Could you check a few things on this model? Use its own coordinates, in mm. Face numbers are marked on the shaded views. A direction names the side the tool comes from. Coordinates: 2 decimals unless noted, no trailing zeros. Order: outer loops, then holes, each group sorted by start corner. A loop starts at its lowest first (then second) coordinate and runs counter-clockwise, first axis right, second up. Notation, with made-up numbers: (88, 76.25) - (107, 76.25) arc R33 ccw to (107, 112.25) - close; hole circle Ø7 at (-0.75, 17). An arc over 180 degrees is marked (long way). Answer as a JSON object with one key per item and string values. Group by question number.
(1) Imagine slicing it at D-D, the plane y = -26.5. Write out the boundary of the cut face in (x, z).
(2) Imagine slicing it at B-B, the plane z = 4.75. Write out the boundary of the cut face in (x, y).
(3) Will these pins go through, and if not, where does the flat tip stop? P1, Ø1.5, axis at x = 68, z = 5.5, coming from the +Y side; P2, Ø2.5, axis at y = -10, z = 3, coming from the -X side; P3, Ø3, axis at y = -25.5, z = 6, coming from the -X side; P4, Ø2.5, axis at x = 75, z = 4, coming from the -Y side.
(4) Imagine slicing it at C-C, the plane x = 35. Write out the boundary of the cut face in (y, z), and give its area (3 significant figures).
(5) We'd pull the mould along X, two halves only. Please class the marked faces 1, 2, 3 and 4: pulls with the +X half, pulls with the -X half, needs draft (parallel to the pull), parting line crosses it, or undercut.
(6) Imagine slicing it at A-A, the plane y = -19.5. Write out the boundary of the cut face in (x, z).
(7) Which directions (+Z, -Z, +X, -X, +Y, -Y) give clear straight access to the entire face, cutting with the end or side of a thin tool? Please do the marked faces 5 and 6.
(8) Please list where these lines run through material, in increasing order: probe 1 along X at (y, z) = (-4, 4.75); probe 2 along X at (y, z) = (-12.5, 2); probe 3 along Y at (x, z) = (30.5, 2.25).
from build123d import *

# Parameters (mm, degrees)
BOSS_EXTRU_1_DEPTH      = 7.5
ESQUISSE2_R             = 1.6
ENL_V_MAT_EXTRU_1_DEPTH = 83.050289457
CHANFREIN1_SIZE         = 8
CHANFREIN1_SIZE2        = 17.156055364
CHANFREIN2_SIZE         = 5
CHANFREIN2_SIZE2        = 10.722534603
ESQUISSE3_W             = 3
ESQUISSE3_H             = 6
ESQUISSE3_H_2           = 5
ENL_V_MAT_EXTRU_2_DEPTH = 83.050289457


with BuildPart() as part:
    # Esquisse1 → Boss.-Extru.1 (new body)
    with BuildSketch(Plane.XY):
        Polygon((0, 0), (0, -30), (76, -30), (76, 0), (55, 0), (55, -23), (14.5, -23), (14.5, 0), align=None)
    extrude(amount=BOSS_EXTRU_1_DEPTH)

    # Esquisse2 → Enlèv. mat.-Extru.1 (cut, through all)
    with BuildSketch(Plane(origin=(0, 0, 0), x_dir=(-1, 0, 0), z_dir=(0, 0, -1))):
        with Locations((-11.746558558, -16.576326178)):
            Circle(ESQUISSE2_R)
        with Locations((-11.746558558, -6.348778822)):
            Circle(ESQUISSE2_R)
        with Locations((-58.966054895, -16.576326178)):
            Circle(ESQUISSE2_R)
        with Locations((-58.966054895, -6.348778822)):
            Circle(ESQUISSE2_R)
    extrude(amount=-ENL_V_MAT_EXTRU_1_DEPTH, mode=Mode.SUBTRACT)

    # Chanfrein1
    chanfrein1_edges = [part.edges().sort_by_distance(p)[0] for p in [
        (0, -30, 3.75),
    ]]
    chanfrein1_side = [part.faces().sort_by_distance(p)[0] for p in [
        (0, -15, 3.75),
    ]]
    chamfer(chanfrein1_edges, length=CHANFREIN1_SIZE, length2=CHANFREIN1_SIZE2, reference=chanfrein1_side[0])

    # Chanfrein2
    chanfrein2_edges = [part.edges().sort_by_distance(p)[0] for p in [
        (76, -30, 3.75),
    ]]
    chanfrein2_side = [part.faces().sort_by_distance(p)[0] for p in [
        (76, -15, 3.75),
    ]]
    chamfer(chanfrein2_edges, length=CHANFREIN2_SIZE, length2=CHANFREIN2_SIZE2, reference=chanfrein2_side[0])

    # Esquisse3 → Enlèv. mat.-Extru.2 (cut, through all)
    with BuildSketch(Plane.XY.offset(7.5)):
        with Locations((74.5, -11)):
            Rectangle(ESQUISSE3_W, ESQUISSE3_H)
        with Locations((1.5, -9.5)):
            Rectangle(ESQUISSE3_W, ESQUISSE3_H_2)
    extrude(amount=-ENL_V_MAT_EXTRU_2_DEPTH, mode=Mode.SUBTRACT)


solid = part.part
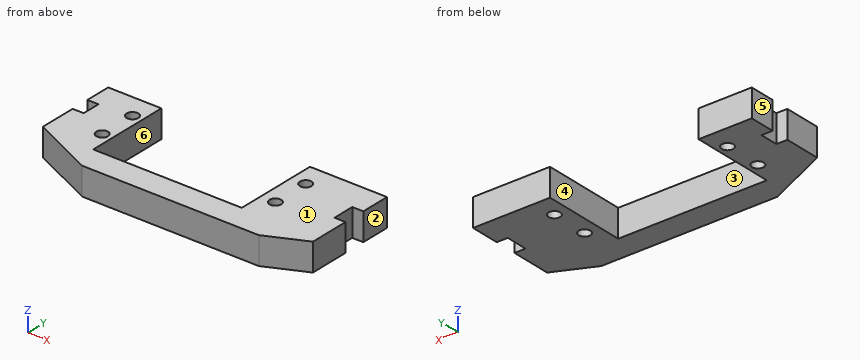
Result set:
{
 "1": {"outline": "(9.65, 0) - (72.78, 0) - (72.78, 7.5) - (9.65, 7.5) - close"},
 "2": {"outline": "(0, -22) - (17.16, -30) - (65.28, -30) - (76, -25) - (76, -14) - (73, -14) - (73, -8) - (76, -8) - (76, 0) - (55, 0) - (55, -23) - (14.5, -23) - (14.5, 0) - (0, 0) - (0, -7) - (3, -7) - (3, -12) - (0, -12) - close; hole circle Ø3.2 at (11.75, -16.58); hole circle Ø3.2 at (11.75, -6.35); hole circle Ø3.2 at (58.97, -16.58); hole circle Ø3.2 at (58.97, -6.35)"},
 "3": {"P1": "stops at y = 0", "P2": "stops at x = 3", "P3": "stops at x = 4.29", "P4": "stops at y = -26.05"},
 "4": {"outline": "(-30, 0) - (-23, 0) - (-23, 7.5) - (-30, 7.5) - close", "area": "52.5 mm^2"},
 "5": {"face 1": "needs draft", "face 2": "pulls with the +X half", "face 3": "undercut", "face 4": "undercut"},
 "6": {"outline": "(0, 0) - (14.5, 0) - (14.5, 7.5) - (0, 7.5) - close; (55, 0) - (76, 0) - (76, 7.5) - (55, 7.5) - close"},
 "7": {"face 5": "+Z, -Z, -X, +Y, -Y", "face 6": "+Z, -Z, +Y"},
 "8": {"probe 1": "x = 0 to 14.5, 55 to 76", "probe 2": "x = 0 to 14.5, 55 to 73", "probe 3": "y = -30 to -23"}
}
